Verification items for the finished model (mm, model axes). Coordinates: 2 decimals unless noted, no trailing zeros. Order: outer loops, then holes, each group sorted by start corner. A loop starts at its lowest first (then second) coordinate and runs counter-clockwise, first axis right, second up. Notation, with made-up numbers: M 44,87 L 60,87 A18 ccw 60,118 Z; hole C 88,-13 d9. An arc over 180 degrees is marked long. Return JSON: item names as keys, results as strings.
```python
from build123d import *

# Parameters (mm, degrees)
SKETCH1_W           = 290
SKETCH1_H           = 150
SKETCH1_R           = 2.875
SKETCH1_R_2         = 12.5
SKETCH1_R_3         = 2.5
BOSS_EXTRUDE2_DEPTH = 5
FILLET1_R           = 10


with BuildPart() as part:
    # Sketch1 → Boss-Extrude2 (new body)
    with BuildSketch(Plane(origin=(0, 0, 0), x_dir=(1, 0, 0), z_dir=(0, 1, 0))):
        Rectangle(SKETCH1_W, SKETCH1_H)
        with Locations((-135.225, 0)):
            Circle(SKETCH1_R, mode=Mode.SUBTRACT)
        with Locations((135.225, 0)):
            Circle(SKETCH1_R, mode=Mode.SUBTRACT)
        with Locations((135.225, 60)):
            Circle(SKETCH1_R, mode=Mode.SUBTRACT)
        with Locations((-135.225, 60)):
            Circle(SKETCH1_R, mode=Mode.SUBTRACT)
        with Locations((-135.225, -60)):
            Circle(SKETCH1_R, mode=Mode.SUBTRACT)
        with Locations((135.225, -60)):
            Circle(SKETCH1_R, mode=Mode.SUBTRACT)
        Circle(SKETCH1_R_2, mode=Mode.SUBTRACT)
        with Locations((-17.5, 17.5)):
            Circle(SKETCH1_R_3, mode=Mode.SUBTRACT)
        with Locations((17.5, 17.5)):
            Circle(SKETCH1_R_3, mode=Mode.SUBTRACT)
        with Locations((17.5, -17.5)):
            Circle(SKETCH1_R_3, mode=Mode.SUBTRACT)
        with Locations((-17.5, -17.5)):
            Circle(SKETCH1_R_3, mode=Mode.SUBTRACT)
    extrude(amount=BOSS_EXTRUDE2_DEPTH)

    # Fillet1
    fillet1_edges = [part.edges().sort_by_distance(p)[0] for p in [
        (-145, 2.5, -75),
        (145, 2.5, -75),
        (145, 2.5, 75),
        (-145, 2.5, 75),
    ]]
    fillet(fillet1_edges, radius=FILLET1_R)


solid = part.part
```
Q1. Go/stop test with a flat-tipped pin: pin 1 (6 mm diameter, centred on x = 17.5, z = -17.5, fed in from -Y). Record where the tip stops, or that it passes through.
Values:
{"pin 1": "y = 0"}
Q2. Cross-section at B-B, the plane x = 0. Record the boundary of the cut face in (y, z).
Values:
{"outline": "M 0,-75 L 5,-75 L 5,-12.5 L 0,-12.5 Z; M 0,12.5 L 5,12.5 L 5,75 L 0,75 Z"}
Q3. Draft check along X on faces 1 (the face through (-2, 5, -18)), 2 (the face through (145, 2, 1)), 3 (the face through (-135.848, 2.465, 62.807)), 4 (the face through (-135.848, 2.465, -57.193)). Enter one of: pulls with the +X half, pulls with the -X half, needs draft (parallel to the pull), parting line crosses it, or undercut.
Values:
{"face 1": "needs draft", "face 2": "pulls with the +X half", "face 3": "undercut", "face 4": "undercut"}
Q4. Cross-section at D-D, the plane z = 0. Record the boundary of the cut face in (x, y), and give its area (3 significant figures).
Values:
{"outline": "M -145,0 L -138.1,0 L -138.1,5 L -145,5 Z; M -132.35,0 L -12.5,0 L -12.5,5 L -132.35,5 Z; M 12.5,0 L 132.35,0 L 132.35,5 L 12.5,5 Z; M 138.1,0 L 145,0 L 145,5 L 138.1,5 Z", "area": "1,270 mm^2"}
Q5. Cross-section at C-C, the plane y = 1.3. State how many separate pieces and enclosed holes the cut face has, and give its area (3 significant figures).
Values:
{"separate pieces": "1", "enclosed holes": "11", "area": "42,700 mm^2"}
Q6. Cross-section at A-A, the plane z = -60. Record the boundary of the cut face in (x, y), and give its area (3 significant figures).
Values:
{"outline": "M -145,0 L -138.1,0 L -138.1,5 L -145,5 Z; M -132.35,0 L 132.35,0 L 132.35,5 L -132.35,5 Z; M 138.1,0 L 145,0 L 145,5 L 138.1,5 Z", "area": "1,390 mm^2"}
Q7. Material ranges on line 1 along X through (y, z) = (1.2, 60); line 2 along Z through (x, y) = (17.5, 1.8); line 3 along X through (y, z) = (1.7, -17.5), recorded low to high.
Values:
{"line 1": "-145 to -138.1, -132.35 to 132.35, 138.1 to 145", "line 2": "-75 to -20, -15 to 15, 20 to 75", "line 3": "-145 to -20, -15 to 15, 20 to 145"}
